For this review, take the finished solid that the model builds, in its own axes (mm). Face numbers are marked on the shaded views. A direction names the side the tool comes from. Give positions to 0.01 mm unless a question says otherwise; leave off trailing zeros. Write each loop counter-clockwise with the first axis right and the second up, starting at its lowest first coordinate (ties: lowest second). Pieces come first, ordered by that corner, then holes. Notation, with made-up numbers: (-30.75, -19) -> (1.25, -19) arc R11 cw to (1.25, -9) -> close; hole circle Ø9 at (39, 23). An arc over 180 degrees is marked (long way). Return JSON: item names as keys, results as strings.
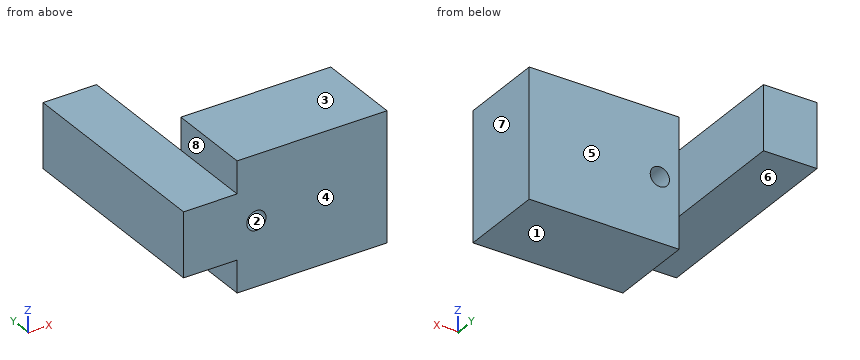
from build123d import *

# Parameters (mm, degrees)
ESQUISSE1_W             = 70
ESQUISSE1_H             = 40
BOSS_EXTRU_1_DEPTH      = 60
ESQUISSE2_R             = 4.5
ENL_V_MAT_EXTRU_1_DEPTH = 60
ESQUISSE3_W             = 30
ESQUISSE3_H             = 40
BOSS_EXTRU_2_DEPTH      = 25
ESQUISSE4_W             = 25
ESQUISSE4_H             = 30
BOSS_EXTRU_3_DEPTH      = 60


with BuildPart() as part:
    # Esquisse1 → Boss.-Extru.1 (new body)
    with BuildSketch(Plane.XY):
        with Locations((-34.135092282, 3.264127517)):
            Rectangle(ESQUISSE1_W, ESQUISSE1_H)
    extrude(amount=BOSS_EXTRU_1_DEPTH)

    # Esquisse2 → Enlèv. mat.-Extru.1 (cut)
    with BuildSketch(Plane(origin=(0, 23.264127517, 0), x_dir=(1, 0, 0), z_dir=(0, 1, 0))):
        with Locations(Location((-60.135092282, -30, 0), (0, 0, 270))):
            Circle(ESQUISSE2_R)
    extrude(amount=-ENL_V_MAT_EXTRU_1_DEPTH, mode=Mode.SUBTRACT)

    # Esquisse3 → Boss.-Extru.2 (add)
    with BuildSketch(Plane.ZY.offset(69.135092282)):
        with Locations((30, 3.264127517)):
            Rectangle(ESQUISSE3_W, ESQUISSE3_H)
    extrude(amount=BOSS_EXTRU_2_DEPTH)

    # Esquisse4 → Boss.-Extru.3 (add)
    with BuildSketch(Plane(origin=(0, 23.264127517, 0), x_dir=(1, 0, 0), z_dir=(0, 1, 0))):
        with Locations((-81.635092282, -30)):
            Rectangle(ESQUISSE4_W, ESQUISSE4_H)
    extrude(amount=BOSS_EXTRU_3_DEPTH)


solid = part.part
1. For pin 1 (12.5 mm diameter, centred on x = -82.5, y = 39, fed in from -Z); pin 2 (9 mm diameter, centred on y = 49.5, z = 22.5, fed in from +X); pin 3 (12 mm diameter, centred on y = 8, z = 54, fed in from -X); pin 4 (16.5 mm diameter, centred on y = -4, z = 9, fed in from -X), all flat-tipped, find the tip position at first contact; note any pin that passes through.
Results found:
{"pin 1": "stops at z = 15", "pin 2": "stops at x = -69.14", "pin 3": "stops at x = -69.14", "pin 4": "stops at x = -94.14"}
2. Add section B-B, the plane y = 21. State the section outline as (x, z) points.
Results found:
{"outline": "(-94.14, 15) -> (-69.14, 15) -> (-69.14, 0) -> (0.86, 0) -> (0.86, 60) -> (-69.14, 60) -> (-69.14, 45) -> (-94.14, 45) -> close; hole circle Ø9 at (-60.14, 30)"}
3. To check wall thickness, follow probe 1 along X at (y, z) = (-2.5, 30); probe 2 along Y at (x, z) = (-21, 39); probe 3 along X at (y, z) = (19.5, 50). State the ranges of each line that lie inside material, in increasing order.
Results found:
{"probe 1": "x = -94.14 to -64.64, -55.64 to 0.86", "probe 2": "y = -16.74 to 23.26", "probe 3": "x = -69.14 to 0.86"}
4. Add section A-A, the plane z = 30. State the section outline as (x, y) points.
Results found:
{"outline": "(-94.14, -16.74) -> (-64.64, -16.74) -> (-64.64, 23.26) -> (-69.14, 23.26) -> (-69.14, 83.26) -> (-94.14, 83.26) -> close; (-55.64, -16.74) -> (0.86, -16.74) -> (0.86, 23.26) -> (-55.64, 23.26) -> close"}
5. Add section D-D, the plane y = 58. State the section outline as (x, z) points.
Results found:
{"outline": "(-94.14, 15) -> (-69.14, 15) -> (-69.14, 45) -> (-94.14, 45) -> close"}
6. For the marked faces 5, 6, 7 and 8, list the 3-axis set-ups (+Z, -Z, +X, -X, +Y, -Y) from which the entire face can be reached by the end or side of a thin tool; tool diameter is ignored.
Results found:
{"face 5": "+Z, -Z, +X, +Y", "face 6": "-Z, -X, +Y, -Y", "face 7": "+Z, -Z, +X, +Y, -Y", "face 8": "+Z, -X, +Y, -Y"}
7. The part is to be moulded in two halves that separate along Z. For the marked faces 1, 2, 3 and 4, say which applies: +Z half, -Z half, draft (parallel to the pull), parting line (faces both ways), or undercut.
Results found:
{"face 1": "-Z half", "face 2": "undercut", "face 3": "+Z half", "face 4": "draft"}
8. Add section C-C, the plane x = -28.5. State the section outline as (y, z) points, plus the area to 3 significant figures.
Results found:
{"outline": "(-16.74, 0) -> (23.26, 0) -> (23.26, 60) -> (-16.74, 60) -> close", "area": "2,400 mm²"}
